Source: CAD feature listing. Evaluate the final solid. Frame: model axes, mm. Face numbers are marked on the shaded views. A direction names the side the tool comes from. Give positions to 0.01 mm unless a question says otherwise; leave off trailing zeros. Write each loop counter-clockwise with the first axis right and the second up, starting at its lowest first coordinate (ties: lowest second). Pieces come first, ordered by that corner, then holes.
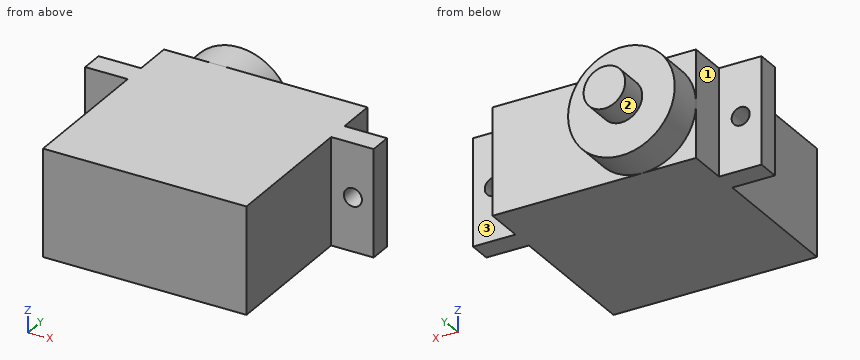
```python
from build123d import *

# Parameters (mm, degrees)
SKETCH1_W           = 4.7
SKETCH1_H           = 2.5
SKETCH1_W_2         = 22.5
SKETCH1_H_2         = 22.7
BOSS_EXTRUDE1_DEPTH = 11.8
SKETCH3_R           = 5.9
BOSS_EXTRUDE2_DEPTH = 4
BOSS_EXTRUDE3_DEPTH = 3.2
SKETCH6_R           = 1
CUT_EXTRUDE1_DEPTH  = 10


with BuildPart() as part:
    # Sketch1 → Boss-Extrude1 (new body)
    with BuildSketch(Plane.XY):
        with Locations((24.85, 17.15)):
            Rectangle(SKETCH1_W, SKETCH1_H)
        with Locations((11.25, 11.35)):
            Rectangle(SKETCH1_W_2, SKETCH1_H_2)
        with Locations((-2.35, 17.15)):
            Rectangle(SKETCH1_W, SKETCH1_H)
    extrude(amount=BOSS_EXTRUDE1_DEPTH)

    # Sketch3 → Boss-Extrude2 (add)
    with BuildSketch(Plane(origin=(0, 22.7, 0), x_dir=(1, 0, 0), z_dir=(0, 1, 0))):
        with Locations((5.9, -5.9)):
            Circle(SKETCH3_R)
    extrude(amount=BOSS_EXTRUDE2_DEPTH)

    # Sketch5 → Boss-Extrude3 (add)
    with BuildSketch(Plane(origin=(0, 26.7, 0), x_dir=(1, 0, 0), z_dir=(0, 1, 0))):
        with BuildLine():
            ThreePointArc((8.2, -5.9), (5.9, -3.6), (3.6, -5.9))
            Line((3.6, -5.9), (8.2, -5.9))
        make_face()
        with BuildLine():
            Line((8.2, -5.9), (3.6, -5.9))
            ThreePointArc((3.6, -5.9), (5.9, -8.2), (8.2, -5.9))
        make_face()
    extrude(amount=BOSS_EXTRUDE3_DEPTH)

    # Sketch6 → Cut-Extrude1 (cut)
    with BuildSketch(Plane(origin=(0, 18.4, 0), x_dir=(1, 0, 0), z_dir=(0, 1, 0))):
        with Locations((24.9, -5.9)):
            Circle(SKETCH6_R)
        with Locations((-2.4, -5.9)):
            Circle(SKETCH6_R)
    extrude(amount=-CUT_EXTRUDE1_DEPTH, mode=Mode.SUBTRACT)


solid = part.part
```
1. Cut plane C-C, the plane y = 3.75. Return the cut outline in (x, z), then the cut area to 4 significant figures.
2. Cut plane B-B, the plane z = 1.75. Return the cut outline in (x, y), then the cut area to 3 significant figures.
3. Cut plane D-D, the plane x = 4.5. Return the cut outline in (y, z).
4. Line query: L1, parallel to X at y = 16.4, z = 5.9; L2, parallel to Z at x = -2.4, y = 17.65; L3, parallel to Y at x = 8.5, z = 6.5. Output: solid intervals per line, ascending.
5. Cut plane A-A, the plane x = 24.9. Return the cut outline in (y, z), then the cut area to 3 significant figures.
6. Access query for the marked faces 1, 2 and 3. Directions: +Z, -Z, +X, -X, +Y, -Y. A direction counts if a zero-diameter tool reaches every point of the face in a straight line with its end or side. Return the directions, or none.
7. Contact query for flat-ended pins moving along their axis: P1, Ø4, axis at x = 25, z = 7, coming from the +Y side; P2, Ø1.6, axis at x = -2.4, z = 5.9, coming from the -Y side; P3, Ø1.4, axis at x = 25, z = 4.5, coming from the -Y side; P4, Ø2, axis at y = 21, z = 8.5, coming from the +X side. Output: stop coordinate, or through.
Response values:
1. outline: (0, 0) - (22.5, 0) - (22.5, 11.8) - (0, 11.8) - close
1. area: 265.5 mm2
2. outline: (-4.7, 15.9) - (0, 15.9) - (0, 0) - (22.5, 0) - (22.5, 15.9) - (27.2, 15.9) - (27.2, 18.4) - (22.5, 18.4) - (22.5, 22.7) - (10.09, 22.7) - (10.09, 26.7) - (1.71, 26.7) - (1.71, 22.7) - (0, 22.7) - (0, 18.4) - (-4.7, 18.4) - close
2. area: 568 mm2
3. outline: (0, 0) - (22.7, 0) - (22.7, 0.17) - (26.7, 0.17) - (26.7, 4.08) - (29.9, 4.08) - (29.9, 7.72) - (26.7, 7.72) - (26.7, 11.63) - (22.7, 11.63) - (22.7, 11.8) - (0, 11.8) - close
4. L1: x = -4.7 to -3.4, -1.4 to 23.9, 25.9 to 27.2
4. L2: z = 0 to 4.9, 6.9 to 11.8
4. L3: y = 0 to 26.7
5. outline: (15.9, 0) - (18.4, 0) - (18.4, 4.9) - (15.9, 4.9) - close; (15.9, 6.9) - (18.4, 6.9) - (18.4, 11.8) - (15.9, 11.8) - close
5. area: 24.5 mm2
6. face 1: +Z, -Z, -X, +Y
6. face 2: +Y
6. face 3: +Z, -Z, +X, +Y
7. P1: stops at y = 18.4
7. P2: passes through
7. P3: stops at y = 15.9
7. P4: stops at x = 22.5
